Verification items for the finished model (mm, model axes). A direction names the side the tool comes from. Round coordinates to 2 decimals unless told otherwise and drop trailing zeros. Write each loop counter-clockwise with the first axis right and the second up, starting at its lowest first coordinate (ties: lowest second). Pieces come first, ordered by that corner, then holes. Notation, with made-up numbers: (-4.75, -10.5) -> (2.25, -10.5) arc R20 ccw to (2.25, 22.5) -> close; hole circle Ø7 at (-19, 12.25). An arc over 180 degrees is marked (long way). Answer as a JSON object with one key per item and string values. Group by question number.
(1) Gauge pin test, flat ends, axial feed: pin 1 Ø5 at (x, y) = (75, 0.5) entering from +Z; pin 2 Ø0.5 at (y, z) = (1, 4.5) entering from +X; pin 3 Ø1.2 at (x, z) = (93, 1) entering from -Y. Record the tip position at first contact, or that the pin passes through.
(2) Set-up check for faces 3 (the face through (-10, 0, 5)), 4 (the face through (93, 0, 4)), 5 (the face through (93, -3, 2)), 6 (the face through (-10, 5, 2)), 7 (the face through (93, 3, 2)): record each of +Z, -Z, +X, -X, +Y, -Y from which the full face is reachable in a straight line by a thin tool's end or side.
(3) Sectioned sample at A-A on y = -0.25. Record the cut outline in (x, z).
(4) Sectioned sample at B-B on z = 2.15. Record the cut outline in (x, y).
(5) Sectioned sample at C-C on x = 175. Record the cut outline in (y, z).
(6) Draft check along X on faces 1 (the face through (-10, -5, 2)), 2 (the face through (-20, 0, 2)). Enter one of: released by +X, released by -X, zero draft, split by the parting line, or undercut.
(7) Scan lines: L1, parallel to Y at x = 115, z = 3.7; L2, parallel to Z at x = 123, y = 0; L3, parallel to X at y = -1.75, z = 3.05. Record each from-to range of solid material in increasing order. Write a range as from..to.
```python
from build123d import *

# Parameters (mm, degrees)
BOX_W        = 190
BOX_H        = 6
BOX_DEPTH    = 4
FILLET001_R  = 1
BOX001_W     = 20
BOX001_H     = 10
BOX001_DEPTH = 5
FILLET_R     = 3


with BuildPart() as handle_fillet:
    # Box → Box (new body)
    with BuildSketch(Plane(origin=(0, -3, 0), x_dir=(1, 0, 0), z_dir=(0, 0, 1))):
        with Locations((95, 3)):
            Rectangle(BOX_W, BOX_H)
    extrude(amount=BOX_DEPTH)

    # Fillet001
    fillet001_edges = [handle_fillet.edges().sort_by_distance(p)[0] for p in [
        (190, -3, 2),
        (190, 0, 4),
        (190, 3, 2),
        (190, 0, 0),
    ]]
    fillet(fillet001_edges, radius=FILLET001_R)


with BuildPart() as spade:
    # Box001 → Box001 (new body)
    with BuildSketch(Plane(origin=(-20, -5, 0), x_dir=(1, 0, 0), z_dir=(0, 0, 1))):
        with Locations((10, 5)):
            Rectangle(BOX001_W, BOX001_H)
    extrude(amount=BOX001_DEPTH)

    # Fillet
    fillet_edges = [spade.edges().sort_by_distance(p)[0] for p in [
        (-20, -5, 2.5),
        (-20, 5, 2.5),
        (0, -5, 2.5),
        (0, 5, 2.5),
    ]]
    fillet(fillet_edges, radius=FILLET_R)

    # Fusion: union handle fillet
    add(handle_fillet.part)


solid = spade.part
```
Computed values:
{
 "1": {"pin 1": "z = 4", "pin 2": "x = 0", "pin 3": "y = -3"},
 "2": {"face 3": "+Z, +X, -X, +Y, -Y", "face 4": "+Z, +X, +Y, -Y", "face 5": "+Z, -Z, +X, -Y", "face 6": "+Z, -Z, +X, -X, +Y", "face 7": "+Z, -Z, +X, +Y"},
 "3": {"outline": "(-20, 0) -> (189, 0) arc R1 ccw to (190, 1) -> (190, 3) arc R1 ccw to (189, 4) -> (0, 4) -> (0, 5) -> (-20, 5) -> close"},
 "4": {"outline": "(-20, -2) arc R3 ccw to (-17, -5) -> (-3, -5) arc R3 ccw to (0, -2) -> (0, -3) -> (189, -3) arc R1 ccw to (190, -2) -> (190, 2) arc R1 ccw to (189, 3) -> (0, 3) -> (0, 2) arc R3 ccw to (-3, 5) -> (-17, 5) arc R3 ccw to (-20, 2) -> close"},
 "5": {"outline": "(-3, 0) -> (3, 0) -> (3, 4) -> (-3, 4) -> close"},
 "6": {"face 1": "zero draft", "face 2": "released by -X"},
 "7": {"L1": "-3..3", "L2": "0..4", "L3": "-20..190"}
}
